```python
from build123d import *

# Parameters (mm, degrees)
SKETCH1_W           = 29.5
SKETCH1_H           = 12
BOSS_EXTRUDE1_DEPTH = 3
BOSS_EXTRUDE7_DEPTH = 12
BOSS_EXTRUDE8_DEPTH = 5
SKETCH16_R          = 1.5
CUT_EXTRUDE11_DEPTH = 24
FILLET5_R           = 2
SKETCH17_OUTSIDE_W  = 67.126
SKETCH17_OUTSIDE_H  = 38.954
SKETCH17_OUTSIDE_R  = 14.75
CUT_EXTRUDE12_DEPTH = 3


with BuildPart() as part:
    # Sketch1 → Boss-Extrude1 (new body)
    with BuildSketch(Plane(origin=(0, 0, 0), x_dir=(1, 0, 0), z_dir=(0, 1, 0))):
        Rectangle(SKETCH1_W, SKETCH1_H)
    extrude(amount=BOSS_EXTRUDE1_DEPTH)



with BuildPart() as body_2:
    # Sketch14 → Boss-Extrude7 (new body, symmetric)
    with BuildSketch(Plane.XY):
        with BuildLine():
            Line((-26.83281573, 13.416407865), (-16, 8))
            Line((-16, 8), (16, 8))
            Line((16, 8), (26.83281573, 13.416407865))
            ThreePointArc((26.83281573, 13.416407865), (0, 30), (-26.83281573, 13.416407865))
        make_face()
    extrude(amount=BOSS_EXTRUDE7_DEPTH, both=True)


with BuildPart() as part_1:
    add(part.part)

    add(body_2.part)  # Boss-Extrude8 merges body 2
    # Sketch15 → Boss-Extrude8 (add)
    with BuildSketch(Plane(origin=(0, 3, 0), x_dir=(-1, 0, 0), z_dir=(0, 1, 0))):
        with BuildLine():
            Line((-9.219544457, 6), (9.219544457, 6))
            ThreePointArc((9.219544457, 6), (11, 0), (9.219544457, -6))
            Line((9.219544457, -6), (-9.219544457, -6))
            ThreePointArc((-9.219544457, -6), (-11, 0), (-9.219544457, 6))
        make_face()
    extrude(amount=BOSS_EXTRUDE8_DEPTH)

    # Sketch16 → Cut-Extrude11 (cut)
    with BuildSketch(Plane(origin=(0, 0, -12), x_dir=(-1, 0, 0), z_dir=(0, 0, -1))):
        with Locations((-23.713219718, 18.376158756)):
            Circle(SKETCH16_R)
        with Locations((-13.204454501, 26.937750117)):
            Circle(SKETCH16_R)
        with Locations((0, 30)):
            Circle(SKETCH16_R)
        with Locations((13.204454501, 26.937750117)):
            Circle(SKETCH16_R)
        with Locations((23.713219718, 18.376158756)):
            Circle(SKETCH16_R)
    extrude(amount=-CUT_EXTRUDE11_DEPTH, mode=Mode.SUBTRACT)

    # Fillet5
    fillet5_edges = [part_1.edges().sort_by_distance(p)[0] for p in [
        (26.83281573, 13.416407865, 0),
        (-21.416407865, 10.708203932, -12),
        (-26.83281573, 13.416407865, 0),
        (0, 8, -12),
        (-16, 8, 0),
        (21.416407865, 10.708203932, -12),
        (16, 8, 0),
        (-21.416407865, 10.708203932, 12),
        (0, 8, 12),
        (21.416407865, 10.708203932, 12),
    ]]
    fillet(fillet5_edges, radius=FILLET5_R)

    # Sketch17 outside → Cut-Extrude12 (cut)
    with BuildSketch(Plane.XZ):
        Rectangle(SKETCH17_OUTSIDE_W, SKETCH17_OUTSIDE_H)
        Circle(SKETCH17_OUTSIDE_R, mode=Mode.SUBTRACT)
    extrude(amount=-CUT_EXTRUDE12_DEPTH, mode=Mode.SUBTRACT)


solid = part_1.part
```
Model file for the job. Use its own axes, mm. A direction names the side the tool comes from. Coordinates: 2 decimals unless noted, no trailing zeros. Order: outer loops, then holes, each group sorted by start corner. A loop starts at its lowest first (then second) coordinate and runs counter-clockwise, first axis right, second up. Notation, with made-up numbers: (24, 60) - (64, 60) arc R19 ccw to (64, 83) - close; hole circle Ø11 at (64, -6). An arc over 180 degrees is marked (long way). Return JSON: item names as keys, results as strings. Group by question number.
1) Flat gauge pins, fed straight in: P1, Ø9, axis at x = 2.5, y = 5, coming from the -Z side; P2, Ø1, axis at x = 10, z = -1, coming from the +Y side; P3, Ø6, axis at x = 12, z = 0.5, coming from the +Y side. Where does each tip first touch, or does it go through?
2) Tool access for faces 4 (the cylindrical face through (14.75, 1.48, -0.09)), 5 (the flat face through (0, 4, -6)), 6 (the cylindrical face through (-21.268, 11.272, 11.399)): list every direction of +Z, -Z, +X, -X, +Y, -Y with a clear straight run to the whole face (end or side of a thin tool).
3) Mould opens along Y. For faces 1 (the flat face through (13, 3, 0)), 2 (the flat face through (0, 18, -12)), 3 (the cylindrical face through (6.85, 29.207, 0.168)) say: released by +Y, released by -Y, zero draft, split by the parting line, or undercut.
4) Saw through at A-A, the plane x = 0. Write the cut outline in (y, z).
5) Saw through at B-B, the plane z = 1.25. Write the cut outline in (x, y), plus the area to 3 significant figures.
6) Saw through at C-C, the plane y = 21.75. Write the cut outline in (x, z), plus the area to 3 significant figures.
7) Probe line 1 (X direction, y = 25.75, z = -4); line 2 (Z direction, x = 8.5, y = 2); line 3 (Y direction, x = -12, z = -0.25). List the from-to ranges inside material, lowest first. Write a range as from..to.
8) Saw through at D-D, the plane z = 3.75. Write the cut outline in (x, y).
Values found:
{
 "1": {"P1": "stops at z = -11.94", "P2": "stops at y = 28.46", "P3": "stops at y = 28.62"},
 "2": {"face 4": "+X, -Y", "face 5": "-Z, +X, -X, -Y", "face 6": "+Z, -X, -Y"},
 "3": {"face 1": "undercut", "face 2": "zero draft", "face 3": "released by +Y"},
 "4": {"outline": "(0, -6) - (8, -6) - (8, -10) arc R2 ccw to (10, -12) - (28.5, -12) - (28.5, 12) - (10, 12) arc R2 ccw to (8, 10) - (8, 6) - (0, 6) - close"},
 "5": {"outline": "(-25.81, 15.3) arc R2 ccw to (-24.98, 12.49) - (-16.42, 8.21) arc R2 ccw to (-15.53, 8) - (-10.93, 8) - (-10.93, 3) - (-14.7, 3) - (-14.7, 0) - (14.7, 0) - (14.7, 3) - (10.93, 3) - (10.93, 8) - (15.53, 8) arc R2 ccw to (16.42, 8.21) - (24.98, 12.49) arc R2 ccw to (25.81, 15.3) arc R30 ccw to (24.6, 17.17) arc R1.5 cw to (22.77, 19.54) arc R30 ccw to (14.53, 26.24) arc R1.5 cw to (11.84, 27.56) arc R30 ccw to (1.5, 29.96) arc R1.5 cw to (-1.5, 29.96) arc R30 ccw to (-11.84, 27.56) arc R1.5 cw to (-14.53, 26.24) arc R30 ccw to (-22.77, 19.54) arc R1.5 cw to (-24.6, 17.17) arc R30 ccw to start", "area": "1,050 mm²"},
 "6": {"outline": "(-20.66, -12) - (20.66, -12) - (20.66, 12) - (-20.66, 12) - close", "area": "992 mm²"},
 "7": {"line 1": "x = -15.39..-14.12, -12.29..12.29, 14.12..15.39", "line 2": "z = -6..6", "line 3": "y = 0..3, 8..26.04"},
 "8": {"outline": "(-25.81, 15.3) arc R2 ccw to (-24.98, 12.49) - (-16.42, 8.21) arc R2 ccw to (-15.53, 8) - (-10.34, 8) - (-10.34, 3) - (-14.27, 3) - (-14.27, 0) - (14.27, 0) - (14.27, 3) - (10.34, 3) - (10.34, 8) - (15.53, 8) arc R2 ccw to (16.42, 8.21) - (24.98, 12.49) arc R2 ccw to (25.81, 15.3) arc R30 ccw to (24.6, 17.17) arc R1.5 cw to (22.77, 19.54) arc R30 ccw to (14.53, 26.24) arc R1.5 cw to (11.84, 27.56) arc R30 ccw to (1.5, 29.96) arc R1.5 cw to (-1.5, 29.96) arc R30 ccw to (-11.84, 27.56) arc R1.5 cw to (-14.53, 26.24) arc R30 ccw to (-22.77, 19.54) arc R1.5 cw to (-24.6, 17.17) arc R30 ccw to start"}
}
